from build123d import *

# Parameters (mm, degrees)
CHAMFER1_SIZE = 0.8


with BuildPart() as part:
    # Sketch1 → Revolve1 (revolve)
    with BuildSketch(Plane.XY, mode=Mode.PRIVATE) as revolve1_sk:
        with BuildLine():
            Line((0, 0), (0, 0.5))
            Line((0, 0.5), (-0.3, 0.5))
            ThreePointArc((-0.3, 0.5), (-1.007106781, 0.792893219), (-1.3, 1.5))
            Line((-1.3, 1.5), (-1.3, 9.45))
            ThreePointArc((-1.3, 9.45), (-1.95, 10.1), (-2.6, 9.45))
            Line((-2.6, 9.45), (-2.6, 1.5))
            Line((-2.6, 1.5), (-4.1, 1.5))
            Line((-4.1, 1.5), (-4.1, 0))
            Line((-4.1, 0), (0, 0))
        make_face()
    revolve(revolve1_sk.sketch.rotate(Axis((0, -1000, 0), (0, 1, 0)), 180), axis=Axis((0, -1000, 0), (0, 1, 0)))

    # Chamfer1
    chamfer1_edges = [part.edges().sort_by_distance(p)[0] for p in [
        (-4.1, 0, 0),
    ]]
    chamfer(chamfer1_edges, length=CHAMFER1_SIZE)


solid = part.part
Check sheet for the modelled part. Datum: model origin and axes. Units: mm. A direction names the side the tool comes from. Round coordinates to 2 decimals unless told otherwise and drop trailing zeros. Loops run counter-clockwise (first coordinate to the right, second up) from the corner with the lowest first, then second, coordinate; pieces in that order, holes last. Notation, with made-up numbers: M -26.75,7.5 L 26.25,7.5 A13 cw 26.25,31.5 Z; hole C -31.5,4.25 d2. An arc over 180 degrees is marked long. One line per item, written item: value.
(1) Thickness scan on line 1 (Y direction, x = -2.75, z = -0.75); line 2 (Z direction, x = 0, y = 3.5); line 3 (Z direction, x = 0.5, y = 7). Record the ranges inside material, lowest first.
Computed values:
line 1: y = 0 to 1.5
line 2: z = -2.6 to -1.3, 1.3 to 2.6
line 3: z = -2.55 to -1.2, 1.2 to 2.55
(2) Sectioned sample at A-A, the plane y = 3. Record the cut outline in (x, z).
Computed values:
outline: C 0,0 d5.2; hole C 0,0 d2.6
(3) Access from +Z, -Z, +X, -X, +Y, -Y to the whole of each face (thin tool, end or side, straight path). Record for faces 4 (the face through (-0.534, 1.145, -4.065)), 5 (the face through (0, 1.5, 3)).
Computed values:
face 4: +Y, -Y
face 5: +Y
(4) Release check for a two-part mould opening along X. For faces 1 (the face through (0, 0, 0)), 2 (the face through (2.48, 5.42, -0.78)), 3 (the face through (1.24, 5.53, -0.39)) record: +X half, -X half, draft (parallel to the pull), parting line (faces both ways), or undercut.
Computed values:
face 1: draft
face 2: parting line
face 3: undercut
(5) Depth check by flat-ended pin: pin 1 Ø1 at (x, y) = (-0.5, 7.5) entering from +Z. Enter the tip coordinate at first touch or a pass-through.
Computed values:
pin 1: stops at z = 2.6
